```python
from build123d import *

# Parameters (mm, degrees)
F0_W     = 73
F0_H     = 38
F0_W_2   = 69
F0_H_2   = 34
F1_DEPTH = 2
F2_DEPTH = 40
F3_R     = 4
F4_DEPTH = 73.001


with BuildPart() as f1:
    # F0 (on Top) → F1 (new body)
    with BuildSketch(Plane.XY):
        Rectangle(F0_W, F0_H)
        Rectangle(F0_W_2, F0_H_2, mode=Mode.SUBTRACT)
        Rectangle(F0_W_2, F0_H_2)
    extrude(amount=F1_DEPTH)

    # F0 (on Top) → F2 (join)
    with BuildSketch(Plane.XY):
        Rectangle(F0_W, F0_H)
        Rectangle(F0_W_2, F0_H_2, mode=Mode.SUBTRACT)
    extrude(amount=-F2_DEPTH)

    # F3 (on face) → F4 (cut, through all)
    with BuildSketch(Plane(origin=(-36.5, 0, 0), x_dir=(0, -1, 0), z_dir=(-1, 0, 0))):
        with Locations((-10.416073, -5.953962)):
            Circle(F3_R)
    extrude(amount=-F4_DEPTH, mode=Mode.SUBTRACT)


solid = f1.part
```
CAD build for the part. Positions are in the model's coordinates, mm. A direction names the side the tool comes from. Round coordinates to 2 decimals unless told otherwise and drop trailing zeros. Order: outer loops, then holes, each group sorted by start corner. A loop starts at its lowest first (then second) coordinate and runs counter-clockwise, first axis right, second up. Notation, with made-up numbers: (82.5, 66) -> (127.5, 66) arc R15 cw to (127.5, 88) -> close; hole circle Ø4 at (44, 66.25). An arc over 180 degrees is marked (long way). Write item = value, one per line.
(1) Cut at B-B (y = 12). Write the cut outline in (x, z), plus the area to 3 significant figures.
Answers follow:
outline = (-36.5, -40) -> (-34.5, -40) -> (-34.5, -9.63) -> (-36.5, -9.63) -> close; (-36.5, -2.28) -> (-34.5, -2.28) -> (-34.5, 0) -> (34.5, 0) -> (34.5, -2.28) -> (36.5, -2.28) -> (36.5, 2) -> (-36.5, 2) -> close; (34.5, -40) -> (36.5, -40) -> (36.5, -9.63) -> (34.5, -9.63) -> close
area = 277 mm²
(2) Pull direction Y, two halves, no side cores. Call faces 3 (the flat face through (-1, 19, -19)), 4 (the flat face through (34.5, 0, -20)), 5 (the flat face through (-3, -18, -40)): +Y half, -Y half, draft (parallel to the pull), parting line (faces both ways), or undercut.
Answers follow:
face_3 = +Y half
face_4 = undercut
face_5 = draft
(3) 3-axis set-ups, long thin cutter, end or side, ignore diameter. For faces 1 (the cylindrical face through (35.486, 14.412, -5.778)), 2 (the flat face through (0, 0, 0)): which of +Z, -Z, +X, -X, +Y, -Y reach the whole face in a straight line?
Answers follow:
face_1 = +X, -X
face_2 = -Z
(4) Drill centre lines: L1, parallel to X at y = 0.5, z = -3; L2, parallel to Y at x = -1.5, z = -1; L3, parallel to Z at x = 20, y = -8.5. Where is each one in solid material? Low to high.
Answers follow:
L1 = -36.5 to -34.5, 34.5 to 36.5
L2 = -19 to -17, 17 to 19
L3 = 0 to 2
(5) Cut at C-C (z = -9). Write the cut outline in (x, y), plus the area to 3 significant figures.
Answers follow:
outline = (-36.5, -19) -> (36.5, -19) -> (36.5, 7.82) -> (34.5, 7.82) -> (34.5, -17) -> (-34.5, -17) -> (-34.5, 7.82) -> (-36.5, 7.82) -> close; (-36.5, 13.01) -> (-34.5, 13.01) -> (-34.5, 17) -> (34.5, 17) -> (34.5, 13.01) -> (36.5, 13.01) -> (36.5, 19) -> (-36.5, 19) -> close
area = 407 mm²
(6) Cut at A-A (z = -31). Write the cut outline in (x, y).
Answers follow:
outline = (-36.5, -19) -> (36.5, -19) -> (36.5, 19) -> (-36.5, 19) -> close; hole (-34.5, -17) -> (34.5, -17) -> (34.5, 17) -> (-34.5, 17) -> close
(7) Cut at D-D (y = -6). Write the cut outline in (x, z).
Answers follow:
outline = (-36.5, -40) -> (-34.5, -40) -> (-34.5, 0) -> (34.5, 0) -> (34.5, -40) -> (36.5, -40) -> (36.5, 2) -> (-36.5, 2) -> close
